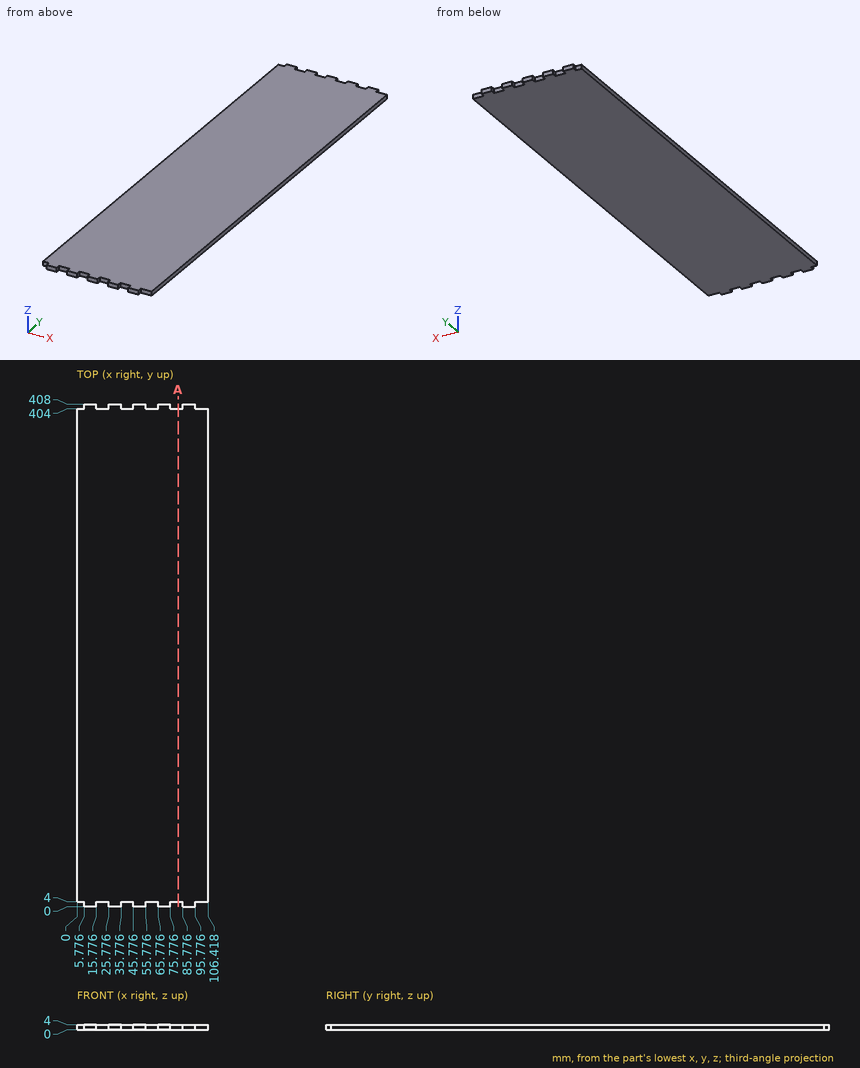
Geometry check sheet. Reference: drawing and pictorial views, mm from the part's lowest x, y, z. Coordinates: 2 decimals unless noted, no trailing zeros. Order: outer loops, then holes, each group sorted by start corner. A loop starts at its lowest first (then second) coordinate and runs counter-clockwise, first axis right, second up.
Item 1: Material ranges on L1, parallel to Y at x = 56, z = 1.25, recorded low to high.
Filled in:
L1: y = 4 to 404
Item 2: Section check A-A, the plane x = 82. Enter the section's corners in (y, z), then the cut area to 3 significant figures.
Filled in:
outline: (4, 0) - (404, 0) - (404, 4) - (4, 4) - close
area: 1,600 mm2
Item 3: Depth check by flat-ended pin: pin 1 (1 mm diameter, centred on x = 26.5, z = 3, fed in from -Y); pin 2 (2 mm diameter, centred on y = 406.5, z = 1, fed in from -X); pin 3 (1.2 mm diameter, centred on x = 3.5, z = 1.5, fed in from -Y); pin 4 (2 mm diameter, centred on y = 406.5, z = 1.5, fed in from +X). Enter the tip coordinate at first touch or a pass-through.
Filled in:
pin 1: stops at y = 0
pin 2: stops at x = 5.78
pin 3: stops at y = 4
pin 4: stops at x = 95.78
